```python
from build123d import *

# Parameters (mm, degrees)
F1_DEPTH = 9.5
F3_DEPTH = 25
F4_R     = 35


with BuildPart() as f1:
    # F0 (on Front) → F1 (new body, symmetric)
    with BuildSketch(Plane.XZ):
        Polygon((-315.4700538379, 200), (-200, 0), (200, 0), (315.4700538379, 200), (223.0940107676, 200), (173.0940107676, 113.3974596216), (155.7735026919, 123.3974596216), (200, 200), (-200, 200), (-155.7735026919, 123.3974596216), (-173.0940107676, 113.3974596216), (-223.0940107676, 200), align=None)
    extrude(amount=F1_DEPTH, both=True)

    # F2 (on face) → F3 (cut)
    with BuildSketch(Plane.XZ.offset(9.5)):
        with BuildLine():
            Line((90, 160), (-90, 160))
            ThreePointArc((-90, 160), (-97.0710678119, 157.0710678119), (-100, 150))
            Line((-100, 150), (-100, 90))
            ThreePointArc((-100, 90), (-97.0710678119, 82.9289321881), (-90, 80))
            Line((-90, 80), (90, 80))
            ThreePointArc((90, 80), (97.0710678119, 82.9289321881), (100, 90))
            Line((100, 90), (100, 150))
            ThreePointArc((100, 150), (97.0710678119, 157.0710678119), (90, 160))
        make_face()
    extrude(amount=-F3_DEPTH, mode=Mode.SUBTRACT)

    # F4
    f4_edges = [f1.edges().sort_by_distance(p)[0] for p in [
        (-315.470054, 0, 200),
        (315.470054, 0, 200),
    ]]
    fillet(f4_edges, radius=F4_R)


solid = f1.part
```
The model under review builds one solid part; all positions refer to its coordinate system, in mm. A direction names the side the tool comes from. Round coordinates to 2 decimals unless told otherwise and drop trailing zeros. Loops run counter-clockwise (first coordinate to the right, second up) from the corner with the lowest first, then second, coordinate; pieces in that order, holes last. Notation, with made-up numbers: (12.5, 68) -> (27.5, 68) arc R22 cw to (27.5, 76) -> close; hole circle Ø10 at (59, 57.25). An arc over 180 degrees is marked (long way). Answer as a JSON object with one key per item and string values. Group by question number.
1) Mouldability with a two-part tool opening along Z and no side actions: class faces 3 (the face through (-178.196, -0.133, 162.235)), 4 (the face through (-4, 9.5, 79)), 5 (the face through (-97.15, -0.13, 83.01)), 6 (the face through (-239, 0, 200)) as released by +Z, released by -Z, zero draft, split by the parting line, or undercut.
2) We need section C-C on z = 38.5. Write out the cut boundary in (x, y), then the cut area to 3 significant figures.
3) For pin 1 Ø9.5 at (y, z) = (2.5, 122) entering from +X; pin 2 Ø4 at (y, z) = (-6, 79.5) entering from -X; pin 3 Ø8 at (y, z) = (-3, 163.5) entering from -X, all flat-tipped, find the tip position at first contact; note any pin that passes through.
4) We need section A-A on y = -3.25. Write out the cut boundary in (x, z).
5) We need section B-B on x = 60. Write out the cut boundary in (y, z).
6) We need section D-D on x = -245. Write out the cut boundary in (y, z), then the cut area to 3 significant figures.
7) For faces 1 (the face through (97.15, -0.13, 156.99)), 2 (the face through (239, 0, 200)), list the 3-axis set-ups (+Z, -Z, +X, -X, +Y, -Y) from which the entire face can be reached by the end or side of a thin tool; tool diameter is ignored.
8) For line 1 (Z direction, x = 49, y = 8.25); line 2 (X direction, y = 4.25, z = 119.5); line 3 (X direction, y = -2, z = 90.5), list the stretches that pass through material, from the lowest coordinate up. Write a range as [from, to].
Result set:
{
 "1": {"face 3": "undercut", "face 4": "zero draft", "face 5": "undercut", "face 6": "released by +Z"},
 "2": {"outline": "(-222.23, -9.5) -> (222.23, -9.5) -> (222.23, 9.5) -> (-222.23, 9.5) -> close", "area": "8,440 mm²"},
 "3": {"pin 1": "x = 273.18", "pin 2": "x = -247.05", "pin 3": "x = -289.85"},
 "4": {"outline": "(-285.16, 147.5) -> (-200, 0) -> (200, 0) -> (285.16, 147.5) arc R35 ccw to (254.85, 200) -> (223.09, 200) -> (173.09, 113.4) -> (155.77, 123.4) -> (200, 200) -> (-200, 200) -> (-155.77, 123.4) -> (-173.09, 113.4) -> (-223.09, 200) -> (-254.85, 200) arc R35 ccw to start; hole (-100, 90) arc R10 ccw to (-90, 80) -> (90, 80) arc R10 ccw to (100, 90) -> (100, 150) arc R10 ccw to (90, 160) -> (-90, 160) arc R10 ccw to (-100, 150) -> close"},
 "5": {"outline": "(-9.5, 0) -> (9.5, 0) -> (9.5, 80) -> (-9.5, 80) -> close; (-9.5, 160) -> (9.5, 160) -> (9.5, 200) -> (-9.5, 200) -> close"},
 "6": {"outline": "(-9.5, 77.94) -> (9.5, 77.94) -> (9.5, 200) -> (-9.5, 200) -> close", "area": "2,320 mm²"},
 "7": {"face 1": "+Y, -Y", "face 2": "+Z, +X, -X, +Y, -Y"},
 "8": {"line 1": "[0, 80], [160, 200]", "line 2": "[-268.99, -176.62], [-162.52, -100], [100, 162.52], [176.62, 268.99]", "line 3": "[-252.25, -100], [100, 252.25]"}
}
